Could you check a few things on this model? Use its own coordinates, in mm. A direction names the side the tool comes from. Round coordinates to 2 decimals unless told otherwise and drop trailing zeros. Loops run counter-clockwise (first coordinate to the right, second up) from the corner with the lowest first, then second, coordinate; pieces in that order, holes last. Notation, with made-up numbers: M 5,67.25 L 42,67.25 A26 cw 42,92.25 Z; hole C 71,52 d9. An arc over 180 degrees is marked long. Answer in a Markdown table with one row per item.
```python
from build123d import *

# Parameters (mm, degrees)
SKETCH1_W           = 25.4
SKETCH1_H           = 19.05
SKETCH1_R           = 2
BOSS_EXTRUDE1_DEPTH = 3.175
SKETCH2_W           = 3.175
SKETCH2_H           = 19.05
BOSS_EXTRUDE2_DEPTH = 25.4
RIB1_REACH          = 44.715
SKETCH3_WALL_W      = 121.181225654
SKETCH3_WALL_H      = 3.175


with BuildPart() as part:
    # Sketch1 → Boss-Extrude1 (new body)
    with BuildSketch(Plane.XY):
        with Locations((-12.7, 0)):
            Rectangle(SKETCH1_W, SKETCH1_H)
        with Locations((-9.525, 0)):
            Circle(SKETCH1_R, mode=Mode.SUBTRACT)
        with Locations((-19.05, 0)):
            Circle(SKETCH1_R, mode=Mode.SUBTRACT)
    extrude(amount=BOSS_EXTRUDE1_DEPTH)

    # Sketch2 → Boss-Extrude2 (add)
    with BuildSketch(Plane.XY.offset(3.175)):
        with Locations((-1.5875, 0)):
            Rectangle(SKETCH2_W, SKETCH2_H)
    extrude(amount=BOSS_EXTRUDE2_DEPTH)

    # Sketch3 wall → Rib1 (add, up to next)
    with BuildSketch(Plane(origin=(-14.2875, 9.525, 15.875), x_dir=(0.658504607869, 0, 0.752576694707), z_dir=(0.752576694707, 0, -0.658504607869)), mode=Mode.PRIVATE) as rib1_sk1:
        with Locations((0, 1.5875)):
            Rectangle(SKETCH3_WALL_W, SKETCH3_WALL_H)
    rib1_tool1 = extrude(rib1_sk1.sketch, amount=RIB1_REACH, mode=Mode.PRIVATE) - part.part
    rib1 = rib1_tool1.solids().sort_by_distance((-14.2875, 9.525, 15.875))[0]
    add(rib1)

    # Mirror1: Rib1 across plane
    add(rib1.mirror(Plane.ZX))


solid = part.part
```
1) Will these pins go through, and if not, where does the flat tip stop? P1, Ø10, axis at y = -4, z = 4, coming from the -X side; P2, Ø5, axis at x = -9.525, y = 0, coming from the +Z side (3 decimals); P3, Ø6, axis at y = -6, z = 10, coming from the -X side; P4, Ø8, axis at y = -1.5, z = 24.5, coming from the -X side (3 decimals).
Computed:
| item | result |
|---|---|
| P1 | stops at x = -25.4 |
| P2 | stops at z = 3.175 |
| P3 | stops at x = -22.04 |
| P4 | stops at x = -3.175 |
2) I want a section at D-D, the plane z = 2.75. Please give me the cut outline in (x, y) (3 decimals), plus the area to 3 significant figures.
Computed:
| item | result |
|---|---|
| outline | M -25.4,-9.525 L 0,-9.525 L 0,9.525 L -25.4,9.525 Z; hole C -19.05,0 d4; hole C -9.525,0 d4 |
| area | 459 mm² |
3) I need wall thicknesses on line 1 (Y direction, x = -19.05, z = 2.05) (3 decimals); line 2 (Y direction, x = -3.75, z = 3.5) (3 decimals); line 3 (X direction, y = -1.75, z = 22.5) (3 decimals). Which ranges of each line are inside material? Lowest first, please.
Computed:
| item | result |
|---|---|
| line 1 | y = -9.525 to -2, 2 to 9.525 |
| line 2 | y = -9.525 to -6.35, 6.35 to 9.525 |
| line 3 | x = -3.175 to 0 |
4) Which directions (+Z, -Z, +X, -X, +Y, -Y) give clear straight access to the entire face, cutting with the end or side of a thin tool? Please do faces 1 (the face through (-13, 0, 0)), 2 (the face through (-11, 6.35, 13)).
Computed:
| item | result |
|---|---|
| face 1 | -Z, +X, -X, +Y, -Y |
| face 2 | +Z, -X |
5) If we mould it in two halves opening along Y, with no side actions, what happens to faces 3 (the face through (-11, -6.35, 13)), 4 (the face through (-2, 0, 28.575)), 5 (the face through (-8, -9.525, 10))? For each: released by +Y, released by -Y, zero draft, split by the parting line, or undercut.
Computed:
| item | result |
|---|---|
| face 3 | undercut |
| face 4 | zero draft |
| face 5 | released by -Y |
6) I want a section at C-C, the plane y = 4. Please give me the cut outline in (x, z) (3 decimals), plus the area to 3 significant figures.
Computed:
| item | result |
|---|---|
| outline | M -25.4,0 L 0,0 L 0,28.575 L -3.175,28.575 L -3.175,3.175 L -25.4,3.175 Z |
| area | 161 mm² |
7) I want a section at B-B, the plane x = -19.05. Please give me the cut outline in (y, z) (3 decimals), plus the area to 3 significant figures.
Computed:
| item | result |
|---|---|
| outline | M -9.525,0 L -2,0 L -2,3.175 L -6.35,3.175 L -6.35,10.432 L -9.525,10.432 Z; M 2,0 L 9.525,0 L 9.525,10.432 L 6.35,10.432 L 6.35,3.175 L 2,3.175 Z |
| area | 93.9 mm² |
8) I want a section at A-A, the plane y = 0. Please give me the cut outline in (x, z) (3 decimals).
Computed:
| item | result |
|---|---|
| outline | M -25.4,0 L -21.05,0 L -21.05,3.175 L -25.4,3.175 Z; M -17.05,0 L -11.525,0 L -11.525,3.175 L -17.05,3.175 Z; M -7.525,0 L 0,0 L 0,28.575 L -3.175,28.575 L -3.175,3.175 L -7.525,3.175 Z |
